from build123d import *

# Parameters (mm, degrees)
SKETCH1_R           = 4
BOSS_EXTRUDE1_DEPTH = 10
SKETCH2_W           = 5
SKETCH2_H           = 80
BOSS_EXTRUDE2_DEPTH = 20
BOSS_EXTRUDE3_START = -10
SKETCH5_R           = 4
BOSS_EXTRUDE3_DEPTH = 2
SKETCH3_R           = 1.5
CUT_EXTRUDE1_DEPTH  = 95.024265485
CUT_EXTRUDE2_DEPTH  = 94.584520622
CHAMFER2_SIZE       = 5
FILLET1_R           = 2
FILLET2_R           = 10
CHAMFER1_SIZE       = 5


with BuildPart() as part:
    # Sketch1 → Boss-Extrude1 (new body)
    with BuildSketch(Plane(origin=(0, 0, 0), x_dir=(1, 0, 0), z_dir=(0, 1, 0))):
        Polygon((0, 0), (0, -80), (44.25, -80), (44.25, -64), (12, -64), (12, -16), (44.25, -16), (44.25, 0), align=None)
        with Locations(Location((39, -8, 0), (0, 0, 270))):
            Circle(SKETCH1_R, mode=Mode.SUBTRACT)
        with Locations(Location((39, -72, 0), (0, 0, 90))):
            Circle(SKETCH1_R, mode=Mode.SUBTRACT)
    extrude(amount=BOSS_EXTRUDE1_DEPTH)

    # Sketch2 → Boss-Extrude2 (add)
    with BuildSketch(Plane(origin=(0, 10, 0), x_dir=(1, 0, 0), z_dir=(0, 1, 0))):
        with Locations((2.5, -40)):
            Rectangle(SKETCH2_W, SKETCH2_H)
    extrude(amount=BOSS_EXTRUDE2_DEPTH)

    # Sketch5 → Boss-Extrude3 (add)
    with BuildSketch(Plane(origin=(0, 10, 0), x_dir=(1, 0, 0), z_dir=(0, 1, 0)).offset(BOSS_EXTRUDE3_START)):
        with Locations(Location((39, -72, 0), (0, 0, 90))):
            Circle(SKETCH5_R)
        with Locations(Location((39, -8, 0), (0, 0, 270))):
            Circle(SKETCH5_R)
    extrude(amount=BOSS_EXTRUDE3_DEPTH)

    # Sketch3 → Cut-Extrude1 (cut, through all)
    with BuildSketch(Plane(origin=(5, 0, 0), x_dir=(0, 0, -1), z_dir=(1, 0, 0))):
        with Locations((-70, 20)):
            Circle(SKETCH3_R)
        with Locations((-40, 20)):
            Circle(SKETCH3_R)
        with Locations((-10, 20)):
            Circle(SKETCH3_R)
    extrude(amount=-CUT_EXTRUDE1_DEPTH, mode=Mode.SUBTRACT)

    # Sketch4 → Cut-Extrude2 (cut, through all)
    with BuildSketch(Plane(origin=(0, 10, 0), x_dir=(1, 0, 0), z_dir=(0, 1, 0))):
        with BuildLine():
            Line((39, -7.5), (44.25, -7.5))
            ThreePointArc((44.25, -7.5), (44.75, -8), (44.25, -8.5))
            Line((44.25, -8.5), (39, -8.5))
            ThreePointArc((39, -8.5), (38.5, -8), (39, -7.5))
        make_face()
        with BuildLine():
            Line((39, -71.5), (44.25, -71.5))
            ThreePointArc((44.25, -71.5), (44.75, -72), (44.25, -72.5))
            Line((44.25, -72.5), (39, -72.5))
            ThreePointArc((39, -72.5), (38.5, -72), (39, -71.5))
        make_face()
    extrude(amount=-CUT_EXTRUDE2_DEPTH, mode=Mode.SUBTRACT)

    # Chamfer2
    chamfer2_edges = [part.edges().sort_by_distance(p)[0] for p in [
        (5, 10, 40),
    ]]
    chamfer(chamfer2_edges, length=CHAMFER2_SIZE)

    # Fillet1
    fillet1_edges = [part.edges().sort_by_distance(p)[0] for p in [
        (44.25, 5, 0),
        (44.25, 5, 16),
        (44.25, 5, 64),
        (44.25, 5, 80),
    ]]
    fillet(fillet1_edges, radius=FILLET1_R)

    # Fillet2
    fillet2_edges = [part.edges().sort_by_distance(p)[0] for p in [
        (12, 5, 16),
        (12, 5, 64),
    ]]
    fillet(fillet2_edges, radius=FILLET2_R)

    # Chamfer1
    chamfer1_edges = [part.edges().sort_by_distance(p)[0] for p in [
        (2.5, 30, 80),
        (2.5, 30, 0),
    ]]
    chamfer(chamfer1_edges, length=CHAMFER1_SIZE)


solid = part.part
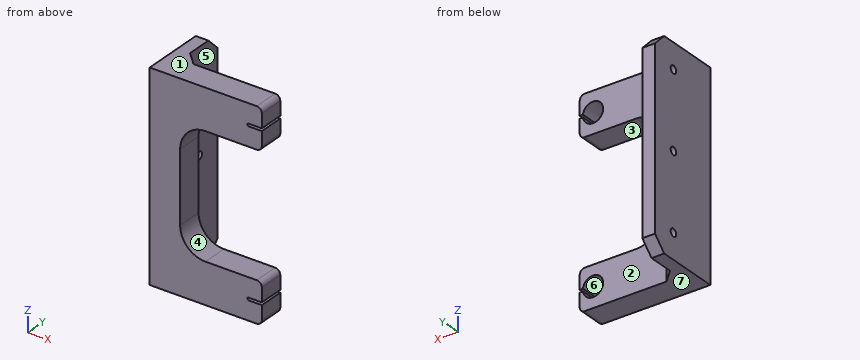
Check sheet for the modelled part. Datum: model origin and axes. Units: mm. Face numbers are marked on the shaded views. A direction names the side the tool comes from. Round coordinates to 2 decimals unless told otherwise and drop trailing zeros. Order: outer loops, then holes, each group sorted by start corner. A loop starts at its lowest first (then second) coordinate and runs counter-clockwise, first axis right, second up. Notation, with made-up numbers: M 34,39 L 42,39 A21 cw 42,54 Z; hole C 15.5,33.25 d5. An arc over 180 degrees is marked long. One line per item, written item: value. Start each with the question number.
1. Release check for a two-part mould opening along Z. For the marked faces 1, 2 and 3 record: released by +Z, released by -Z, zero draft, split by the parting line, or undercut.
2. Access from +Z, -Z, +X, -X, +Y, -Y to the whole of each face (thin tool, end or side, straight path). Record for the marked faces 4, 5, 6 and 7.
3. Gauge pin test, flat ends, axial feed: P1, Ø2, axis at x = 30.5, z = 64.5, coming from the +Y side; P2, Ø4, axis at y = 9, z = 31, coming from the +X side; P3, Ø5, axis at x = 39, z = 8, coming from the +Y side. Record the tip position at first contact, or that the pin passes through.
4. Section check A-A on x = 25. Enter the section's corners in (y, z).
5. Section check C-C on z = 40. Enter the section's corners in (x, y).
6. Scan lines: line 1 along Z through (x, y) = (39, 7.5); line 2 along Y through (x, z) = (2.85, 40); line 3 along Z through (x, y) = (33.5, 2.25). Record each from-to range of solid material in increasing order.
7. Section check B-B on y = 8.5. Enter the section's corners in (x, z), and give its area (3 significant figures).
8. Section check D-D on y = 20. Enter the section's corners in (x, z).
Results found:
1. face 1: released by +Z
1. face 2: zero draft
1. face 3: undercut
2. face 4: +X, +Y, -Y
2. face 5: +Z, -Z, +X, +Y
2. face 6: +Y
2. face 7: -Z, +X, -X, +Y, -Y
3. P1: y = 10
3. P2: x = 12
3. P3: y = 2
4. outline: M 0,0 L 10,0 L 10,16 L 0,16 Z; M 0,64 L 10,64 L 10,80 L 0,80 Z
5. outline: M 0,0 L 12,0 L 12,10 L 10,10 L 5,15 L 5,18.5 L 0,18.5 Z; M 0,21.5 L 5,21.5 L 5,30 L 0,30 Z
6. line 1: 0 to 4, 12 to 16, 64 to 68, 76 to 80
6. line 2: 0 to 18.5, 21.5 to 30
6. line 3: 0 to 16, 64 to 80
7. outline: M 0,0 L 42.25,0 A2 ccw 44.25,2 L 44.25,7.5 L 42.97,7.5 A4 cw long 42.97,8.5 L 44.25,8.5 L 44.25,14 A2 ccw 42.25,16 L 22,16 A10 cw 12,26 L 12,54 A10 cw 22,64 L 42.25,64 A2 ccw 44.25,66 L 44.25,71.5 L 42.97,71.5 A4 cw long 42.97,72.5 L 44.25,72.5 L 44.25,78 A2 ccw 42.25,80 L 0,80 Z
7. area: 1,930 mm^2
8. outline: M 0,0 L 5,0 L 5,8.5 L 0,8.5 Z; M 0,11.5 L 5,11.5 L 5,38.5 L 0,38.5 Z; M 0,41.5 L 5,41.5 L 5,68.5 L 0,68.5 Z; M 0,71.5 L 5,71.5 L 5,80 L 0,80 Z
